Geometry: see drawing. Coordinates: mm, zero at the bounding-box minimum. A direction names the side the tool comes from. Coordinates: 2 decimals unless noted, no trailing zeros. Loops run counter-clockwise (first coordinate to the right, second up) from the corner with the lowest first, then second, coordinate; pieces in that order, holes last. Notation, with made-up numbers: (38.5, 82.25) - (89.5, 82.25) arc R24 cw to (89.5, 108.25) - close; hole circle Ø4 at (42.25, 37.5). An arc over 180 degrees is marked (long way). Use a Markdown table: item, result. Add a question column.
1. Access query for the marked faces 1, 2, 3, 4 and 5. Directions: +Z, -Z, +X, -X, +Y, -Y. A direction counts if a zero-diameter tool reaches every point of the face in a straight line with its end or side. Return the directions, or none.
2. Draft query along X for the marked faces 6, 7, 8 and 9. Return one class per face: released by +X, released by -X, zero draft, split by the parting line, or undercut.
3. Section query A-A on z = 31. Return the cut outline in (x, y).
4. Section query B-B on y = 23.25. Return the cut outline in (x, z), then the cut area to 3 significant figures.
5. Ray query, L1, parallel to Z at x = 13, y = 16; L2, parallel to X at y = 19.25, z = 11; L3, parallel to X at y = 19.5, z = 2. Return the intervals inside material, ascending. Write a range as [from, to].
6. Contact query for flat-ended pins moving along their axis: P1, Ø10, axis at y = 20, z = 33.5, coming from the -X side; P2, Ø9, axis at y = 14.5, z = 27, coming from the +X side; P3, Ø5.5, axis at x = 12.5, y = 18, coming from the -Z side. Output: stop coordinate, or through.
7. Section query D-D on y = 3.5. Return the cut outline in (x, z), then the cut area to 3 significant figures.
8. Section query C-C on x = 55. Return the cut outline in (y, z), then the cut area to 3 significant figures.
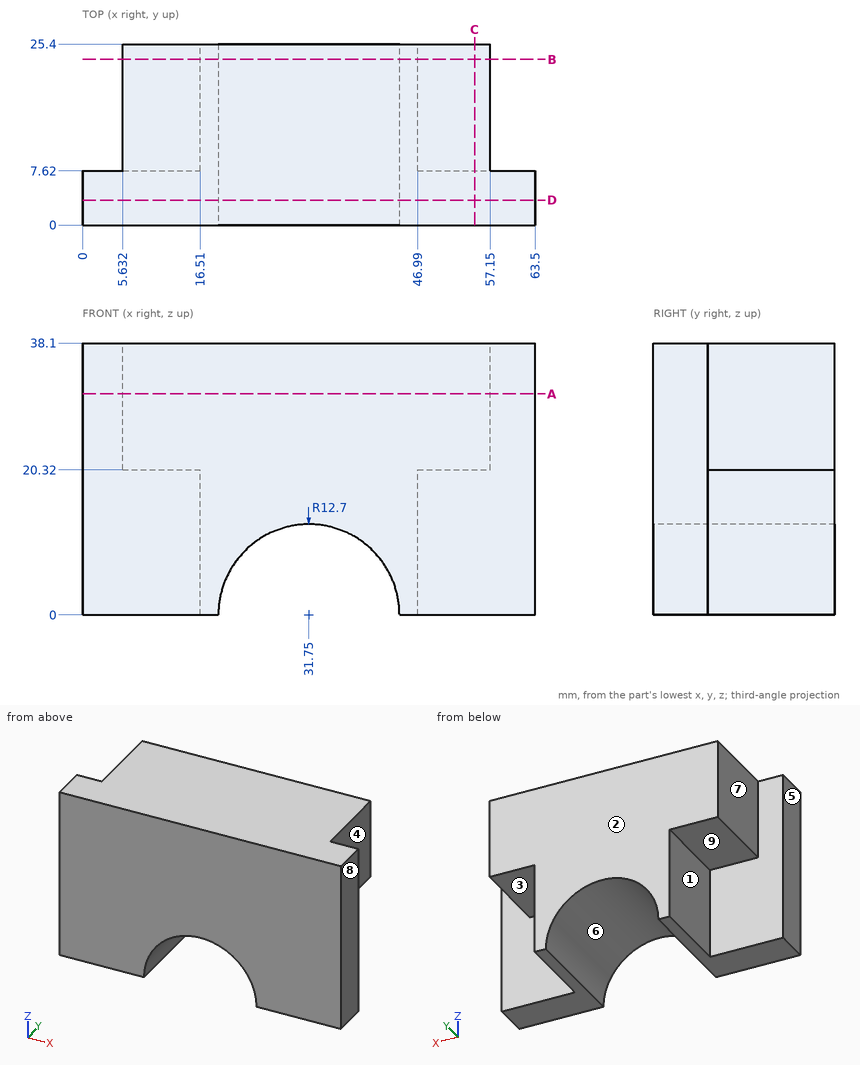
Resolved:
| question | item | result |
|---|---|---|
| 1 | face 1 | -Z, -X, +Y |
| 1 | face 2 | +Z, -Z, +X, -X, +Y |
| 1 | face 3 | -Z, +X, +Y |
| 1 | face 4 | +Z, -Z, +X, +Y |
| 1 | face 5 | +Z, -Z, -X, +Y, -Y |
| 2 | face 6 | undercut |
| 2 | face 7 | released by -X |
| 2 | face 8 | released by +X |
| 2 | face 9 | zero draft |
| 3 | outline | (0, 0) - (63.5, 0) - (63.5, 7.62) - (57.15, 7.62) - (57.15, 25.4) - (5.63, 25.4) - (5.63, 7.62) - (0, 7.62) - close |
| 4 | outline | (5.63, 20.32) - (16.51, 20.32) - (16.51, 0) - (19.05, 0) arc R12.7 cw to (44.45, 0) - (46.99, 0) - (46.99, 20.32) - (57.15, 20.32) - (57.15, 38.1) - (5.63, 38.1) - close |
| 4 | area | 1,280 mm² |
| 5 | L1 | [20.32, 38.1] |
| 5 | L2 | [16.51, 25.4], [38.1, 46.99] |
| 5 | L3 | [16.51, 19.21], [44.29, 46.99] |
| 6 | P1 | x = 5.63 |
| 6 | P2 | x = 57.15 |
| 6 | P3 | z = 20.32 |
| 7 | outline | (0, 0) - (19.05, 0) arc R12.7 cw to (44.45, 0) - (63.5, 0) - (63.5, 38.1) - (0, 38.1) - close |
| 7 | area | 2,170 mm² |
| 8 | outline | (0, 0) - (7.62, 0) - (7.62, 20.32) - (25.4, 20.32) - (25.4, 38.1) - (0, 38.1) - close |
| 8 | area | 606 mm² |
